Source: CAD feature listing. Evaluate the final solid. Frame: model axes, mm. A direction names the side the tool comes from. Coordinates: 2 decimals unless noted, no trailing zeros. Order: outer loops, then holes, each group sorted by start corner. A loop starts at its lowest first (then second) coordinate and runs counter-clockwise, first axis right, second up.
```python
from build123d import *

# Parameters (mm, degrees)
SKETCH_W      = 12.2
SKETCH_H      = 137
PAD_DEPTH     = 29.5
SKETCH002_W   = 27.2
SKETCH002_H   = 166
PAD001_DEPTH  = 2
SKETCH003_W   = 6.5
SKETCH003_H   = 9
PAD002_DEPTH  = 6
SKETCH001_W   = 8.5
SKETCH001_H   = 45.5
SKETCH001_W_2 = 10.5
POCKET_DEPTH  = 25
CHAMFER_SIZE  = 1.5
FILLET_R      = 0.4


with BuildPart() as part:
    # Sketch → Pad (new body)
    with BuildSketch(Plane.XY):
        with Locations((6.1, 68.5)):
            Rectangle(SKETCH_W, SKETCH_H)
    extrude(amount=PAD_DEPTH)

    # Sketch002 → Pad001 (join)
    with BuildSketch(Plane.XY.offset(29.5)):
        with Locations((6.1, 68.73)):
            Rectangle(SKETCH002_W, SKETCH002_H)
    extrude(amount=PAD001_DEPTH)

    # Sketch003 → Pad002 (join)
    with BuildSketch(Plane.XY.offset(29.5)):
        with Locations((6.1, -4.5)):
            Rectangle(SKETCH003_W, SKETCH003_H)
        with Locations((6.1, 141.5)):
            Rectangle(SKETCH003_W, SKETCH003_H)
    extrude(amount=-PAD002_DEPTH)

    # Sketch001 → Pocket (cut)
    with BuildSketch(Plane.XY.offset(31.5)):
        with Locations((7.95, 37.75)):
            Rectangle(SKETCH001_W, SKETCH001_H)
        with Locations((7, 118.25)):
            Rectangle(SKETCH001_W_2, SKETCH001_H)
    extrude(amount=-POCKET_DEPTH, mode=Mode.SUBTRACT)

    # Chamfer
    chamfer_edges = [part.edges().sort_by_distance(p)[0] for p in [
        (6.1, 151.73, 31.5),
        (-7.5, 68.73, 31.5),
        (19.7, 68.73, 31.5),
        (6.1, -14.27, 31.5),
    ]]
    chamfer(chamfer_edges, length=CHAMFER_SIZE)

    # Fillet
    fillet_edges = [part.edges().sort_by_distance(p)[0] for p in [
        (3.7, 37.75, 31.5),
        (7.95, 60.5, 31.5),
        (12.2, 37.75, 31.5),
        (7.95, 15, 31.5),
        (12.25, 118.25, 31.5),
        (7, 95.5, 31.5),
        (1.75, 118.25, 31.5),
        (7, 141, 31.5),
        (12.2, 68.5, 0),
        (0, 68.5, 0),
        (6.1, 137, 0),
        (6.1, 0, 0),
        (12.2, 137, 3.25),
        (0, 137, 14.75),
        (0, 0, 14.75),
        (12.2, 0, 14.75),
        (9.35, -4.5, 23.5),
        (6.1, -9, 23.5),
        (2.85, -4.5, 23.5),
        (2.85, -9, 26.5),
        (9.35, -9, 26.5),
        (12.2, 15, 18),
        (12.2, 37.75, 6.5),
        (12.2, 60.5, 18),
        (12.2, 95.5, 18),
        (12.2, 116.25, 6.5),
        (6.975, 137, 6.5),
        (2.85, 146, 26.5),
        (9.35, 146, 26.5),
        (9.35, 143.5, 23.5),
        (6.1, 146, 23.5),
        (2.85, 143.5, 23.5),
        (6.1, 141, 23.5),
        (9.35, 141, 26.5),
        (2.85, 141, 26.5),
        (1.75, 137, 18),
    ]]
    fillet(fillet_edges, radius=FILLET_R)


solid = part.part
```
Q1. Section query A-A on y = 53. Output: boundary loops of the cut face in (x, z).
Solutions:
outline: (-7.5, 29.5) - (0, 29.5) - (0, 0.4) arc R0.4 ccw to (0.4, 0) - (11.8, 0) arc R0.4 ccw to (12.2, 0.4) - (12.2, 6.1) arc R0.4 ccw to (11.8, 6.5) - (3.7, 6.5) - (3.7, 31.1) arc R0.4 ccw to (3.3, 31.5) - (-6, 31.5) - (-7.5, 30) - close; (12.2, 29.5) - (19.7, 29.5) - (19.7, 30) - (18.2, 31.5) - (12.6, 31.5) arc R0.4 ccw to (12.2, 31.1) - close
Q2. Set-up query: faces 1 (the flat face through (6, -9, 27)), 2 (the flat face through (1.75, 118, 19)), 3 (the flat face through (5, 137, 5)), 4 (the flat face through (9.35, 143, 27)). Return all of +Z, -Z, +X, -X, +Y, -Y with unobstructed straight access to the full face (end or side cutting, diameter ignored); none if empty.
Solutions:
face 1: -Z, +X, -X, -Y
face 2: +Z
face 3: -Z, +X, -X, +Y
face 4: -Z, +X, +Y
Q3. Section query D-D on x = 16. Output: boundary loops of the cut face in (y, z), plus the area to 3 significant figures.
Solutions:
outline: (-14.27, 29.5) - (151.73, 29.5) - (151.73, 30) - (150.23, 31.5) - (-12.77, 31.5) - (-14.27, 30) - close
area: 330 mm2
Q4. Material intervals for line 1 along Y through (x, z) = (5, 26.5); line 2 along Y through (x, z) = (4.5, 12); line 3 along Y through (x, z) = (4, 6), sorted ascending.
Solutions:
line 1: y = -9 to 15, 60.5 to 95.5, 141 to 146
line 2: y = 0 to 15, 60.5 to 95.5
line 3: y = 0 to 137
Q5. Section query C-C on z = 15.5. Output: boundary loops of the cut face in (x, y), plus the area to 3 significant figures.
Solutions:
outline: (0, 0.4) arc R0.4 ccw to (0.4, 0) - (11.8, 0) arc R0.4 ccw to (12.2, 0.4) - (12.2, 14.6) arc R0.4 ccw to (11.8, 15) - (3.7, 15) - (3.7, 60.5) - (11.8, 60.5) arc R0.4 ccw to (12.2, 60.9) - (12.2, 95.1) arc R0.4 ccw to (11.8, 95.5) - (1.75, 95.5) - (1.75, 136.6) arc R0.4 ccw to (1.35, 137) - (0.4, 137) arc R0.4 ccw to (0, 136.6) - close
area: 851 mm2
Q6. Pin query (flat end, axial travel): P1, Ø5, axis at x = 7, y = 116.5, coming from the +Z side; P2, Ø9.5, axis at x = 8, z = 21.5, coming from the +Y side; P3, Ø2, axis at x = 7.5, z = 26, coming from the -Y side. Return the tip coordinate at first contact, or that it passes through.
Solutions:
P1: stops at z = 6.5
P2: stops at y = 146
P3: stops at y = -9
Q7. Pull-direction query (X, two-part tool) for faces 5 (the flat face through (12.2, 68, 12)), 6 (the flat face through (8, 38, 6.5)), 7 (the flat face through (6, 141, 28)), 8 (the flat face through (2.85, -4, 27)); classes: pulls with the +X half, pulls with the -X half, needs draft (parallel to the pull), parting line crosses it, or undercut.
Solutions:
face 5: pulls with the +X half
face 6: needs draft
face 7: undercut
face 8: pulls with the -X half
